from build123d import *

# Parameters (mm, degrees)
ESQUISSE1_R             = 9.875
BOSS_EXTRU_1_DEPTH      = 2
ESQUISSE2_R             = 6.15
BOSS_EXTRU_2_DEPTH      = 6.4
ESQUISSE3_R             = 3.675
BOSS_EXTRU_3_DEPTH      = 22
ENL_V_START             = -22
ENL_V_MAT_EXTRU_1_DEPTH = 22
ESQUISSE5_R             = 1.2
ENL_V_MAT_EXTRU_2_DEPTH = 32.647926472
CONG_1_R                = 1.5


with BuildPart() as part:
    # Esquisse1 → Boss.-Extru.1 (new body)
    with BuildSketch(Plane.XY):
        Circle(ESQUISSE1_R)
    extrude(amount=BOSS_EXTRU_1_DEPTH)

    # Esquisse2 → Boss.-Extru.2 (add)
    with BuildSketch(Plane.XY.offset(2)):
        Circle(ESQUISSE2_R)
    extrude(amount=BOSS_EXTRU_2_DEPTH)

    # Esquisse3 → Boss.-Extru.3 (add)
    with BuildSketch(Plane.XY.offset(8.4)):
        Circle(ESQUISSE3_R)
    extrude(amount=BOSS_EXTRU_3_DEPTH)

    # Esquisse4 → Enlèv. mat.-Extru.1 (cut)
    with BuildSketch(Plane.XY.offset(30.4).offset(ENL_V_START)):
        with BuildLine():
            Line((-2.886173938, -2.275), (2.886173938, -2.275))
            ThreePointArc((2.886173938, -2.275), (0, -3.675), (-2.886173938, -2.275))
        make_face()
    extrude(amount=ENL_V_MAT_EXTRU_1_DEPTH, mode=Mode.SUBTRACT)

    # Esquisse5 → Enlèv. mat.-Extru.2 (cut, through all)
    with BuildSketch(Plane.XY.offset(2)):
        with Locations((0, 8.045346172)):
            Circle(ESQUISSE5_R)
        with Locations((0, -8.054653828)):
            Circle(ESQUISSE5_R)
        with Locations((-8.05, 0)):
            Circle(ESQUISSE5_R)
        with Locations((8.05, 0)):
            Circle(ESQUISSE5_R)
    extrude(amount=-ENL_V_MAT_EXTRU_2_DEPTH, mode=Mode.SUBTRACT)

    # Congé1
    cong_1_edges = [part.edges().sort_by_distance(p)[0] for p in [
        (0, 3.675, 8.4),
        (0, -2.275, 8.4),
    ]]
    fillet(cong_1_edges, radius=CONG_1_R)


solid = part.part
For this review, take the finished solid that the model builds, in its own axes (mm). A direction names the side the tool comes from. Round coordinates to 2 decimals unless told otherwise and drop trailing zeros. Write each loop counter-clockwise with the first axis right and the second up, starting at its lowest first coordinate (ties: lowest second). Pieces come first, ordered by that corner, then holes. Notation, with made-up numbers: (-40, -37.75) -> (9, -37.75) arc R15 ccw to (9, -12.75) -> close; hole circle Ø1 at (13, 39). An arc over 180 degrees is marked (long way). Put each result on its own line as item: value.
Q1. Consider section B-B on x = 0. State the section outline as (y, z) points (3 decimals).
Determined:
outline: (-9.875, 0) -> (-9.255, 0) -> (-9.255, 2) -> (-9.875, 2) -> close; (-6.855, 0) -> (6.845, 0) -> (6.845, 2) -> (6.15, 2) -> (6.15, 8.4) -> (5.175, 8.4) arc R1.5 cw to (3.675, 9.9) -> (3.675, 30.4) -> (-2.275, 30.4) -> (-2.275, 9.9) arc R1.5 cw to (-3.775, 8.4) -> (-6.15, 8.4) -> (-6.15, 2) -> (-6.855, 2) -> close; (9.245, 0) -> (9.875, 0) -> (9.875, 2) -> (9.245, 2) -> close
Q2. To check wall thickness, follow L1, parallel to Y at x = 0, z = 1.5 (3 decimals); L2, parallel to Z at x = 0, y = -5.75; L3, parallel to Z at x = 3, y = -6.75. State the ranges of each line that lie inside material, in increasing order. Write a range as [from, to].
Determined:
L1: y = [-9.875, -9.255], [-6.855, 6.845], [9.245, 9.875]
L2: z = [0, 8.4]
L3: z = [0, 2]
Q3. Machinability: for faces 4 (the cylindrical face through (-1.333, -6.004, 5.155)), 5 (the cylindrical face through (-0.26, -9.226, 1.014)), which of the approach directions +Z, -Z, +X, -X, +Y, -Y give a long, thin tool a straight path to every point of the face, cutting with its end or side? Answer none if there is none.
Determined:
face 4: +Z
face 5: +Z, -Z
Q4. Consider section C-C on x = -8.5. State the section outline as (y, z) points.
Determined:
outline: (-5.03, 0) -> (-1.11, 0) -> (-1.11, 2) -> (-5.03, 2) -> close; (1.11, 0) -> (5.03, 0) -> (5.03, 2) -> (1.11, 2) -> close
Q5. The part is to be moulded in two halves that separate along X. For faces 1 (the flat face through (0, -2.275, 20)), 2 (the cylindrical face through (-7.28, 6.67, 0.99)), 3 (the cylindrical face through (-9.25, 0.05, 1.01)), say which applies: released by +X, released by -X, zero draft, split by the parting line, or undercut.
Determined:
face 1: zero draft
face 2: split by the parting line
face 3: undercut
Q6. Consider section A-A on y = 0. State the section outline as (x, z) points (3 decimals).
Determined:
outline: (-9.875, 0) -> (-9.25, 0) -> (-9.25, 2) -> (-9.875, 2) -> close; (-6.85, 0) -> (6.85, 0) -> (6.85, 2) -> (6.15, 2) -> (6.15, 8.4) -> (5.175, 8.4) arc R1.5 cw to (3.675, 9.9) -> (3.675, 30.4) -> (-3.675, 30.4) -> (-3.675, 9.9) arc R1.5 cw to (-5.175, 8.4) -> (-6.15, 8.4) -> (-6.15, 2) -> (-6.85, 2) -> close; (9.25, 0) -> (9.875, 0) -> (9.875, 2) -> (9.25, 2) -> close
Q7. Clearance check with flat-ended pins moving along their axes: pin 1 Ø3 at (x, z) = (3.5, 7.5) entering from +Y; pin 2 Ø6.5 at (x, z) = (-1, 21) entering from -Y (3 decimals); pin 3 Ø8 at (x, z) = (6, 18.5) entering from +Y. State where each tip first meets the part, or that it passes through.
Determined:
pin 1: stops at y = 5.82
pin 2: stops at y = -2.275
pin 3: stops at y = 3.08
